Source: CAD feature listing. Evaluate the final solid. Frame: model axes, mm. Face numbers are marked on the shaded views. A direction names the side the tool comes from. Coordinates: 2 decimals unless noted, no trailing zeros. Write each loop counter-clockwise with the first axis right and the second up, starting at its lowest first coordinate (ties: lowest second). Pieces come first, ordered by that corner, then holes. Notation, with made-up numbers: (79.25, -14) -> (103.25, -14) arc R26 cw to (103.25, 3) -> close; hole circle Ø11 at (70, 2.25). An arc over 180 degrees is marked (long way). One line per item, written item: value. Start each with the question number.
1. Section query A-A, the plane z = 1.5. Output: boundary loops of the cut face in (x, y).
2. Access query for the marked faces 1 and 2. Directions: +Z, -Z, +X, -X, +Y, -Y. A direction counts if a zero-diameter tool reaches every point of the face in a straight line with its end or side. Return the directions, or none.
3. First-contact query: P1, Ø3, axis at y = 1, z = 6.5, coming from the +X side. Flat tip, straight axial feed; report the tip coordinate or a pass-through.
4. Section query B-B, the plane y = 3.5. Output: boundary loops of the cut face in (x, z), and give its area (3 significant figures).
5. Section query D-D, the plane z = 12. Output: boundary loops of the cut face in (x, y).
6. Line query: line 1 (X direction, y = 6.25, z = 13.25); line 2 (Z direction, x = 16.25, y = 7); line 3 (Z direction, x = 10.5, y = 9.25). Output: solid intervals per line, ascending.
7. Section query C-C, the plane x = 11.5. Output: boundary loops of the cut face in (y, z).
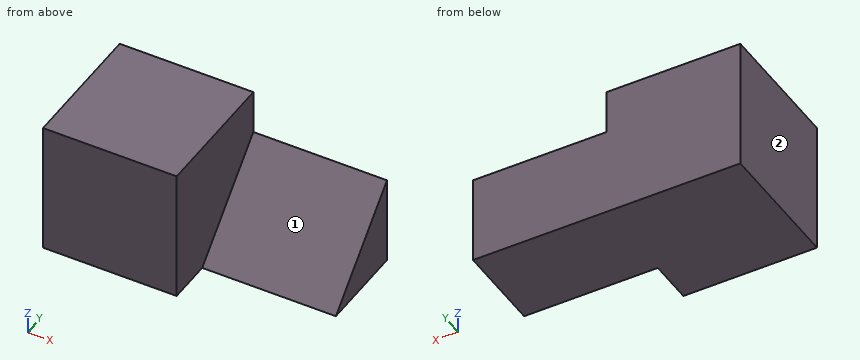
from build123d import *

# Parameters (mm, degrees)
F0_W     = 15
F0_H     = 15
F1_DEPTH = 15
F3_DEPTH = 15


with BuildPart() as f1:
    # F0 (on Top) → F1 (new body)
    with BuildSketch(Plane.XY):
        with Locations((2.898159, 3.825012)):
            Rectangle(F0_W, F0_H)
    extrude(amount=F1_DEPTH)

    # F2 (on face) → F3 (join)
    with BuildSketch(Plane.YZ.offset(10.398159)):
        Polygon((11.325012, 10), (1.325012, 0), (11.325012, 0), align=None)
    extrude(amount=F3_DEPTH)


solid = f1.part
Computed values:
1. outline: (-4.6, -3.67) -> (10.4, -3.67) -> (10.4, 2.83) -> (25.4, 2.83) -> (25.4, 11.33) -> (-4.6, 11.33) -> close
2. face 1: +Z, +X, -Y
2. face 2: +Z, -Z, -X, +Y, -Y
3. P1: stops at x = 10.4
4. outline: (-4.6, 0) -> (25.4, 0) -> (25.4, 2.17) -> (10.4, 2.17) -> (10.4, 15) -> (-4.6, 15) -> close
4. area: 258 mm²
5. outline: (-4.6, -3.67) -> (10.4, -3.67) -> (10.4, 11.33) -> (-4.6, 11.33) -> close
6. line 1: x = -4.6 to 10.4
6. line 2: z = 0 to 5.67
6. line 3: z = 0 to 7.92
7. outline: (1.33, 0) -> (11.33, 0) -> (11.33, 10) -> close
